Design review of the part built by this model. Coordinates are the model's own, in mm. Face numbers are marked on the shaded views. A direction names the side the tool comes from. Give positions to 0.01 mm unless a question says otherwise; leave off trailing zeros. Loops run counter-clockwise (first coordinate to the right, second up) from the corner with the lowest first, then second, coordinate; pieces in that order, holes last.
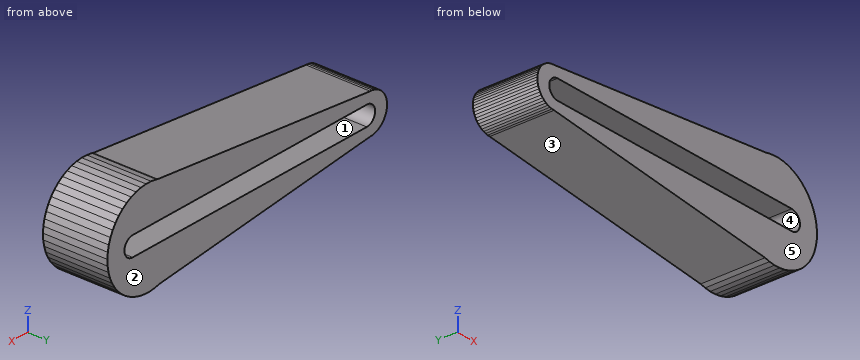
from build123d import *

# Parameters (mm, degrees)
F1_DEPTH = 25.4
F2_W     = 107.95
F2_H     = 7.62
F3_DEPTH = 25.4


with BuildPart() as f1:
    # F0 (on Front) → F1 (new body)
    with BuildSketch(Plane.XZ):
        Polygon((34.795007, 14.206795), (36.671421, 15.617947), (38.709903, 16.782795), (40.878305, 17.682968), (42.411124, 18.103591), (-55.535455, 7.733652), (-54.566239, 7.671582), (-53.612446, 7.488527), (-52.689117, 7.187373), (-51.810813, 6.77287), (-50.991386, 6.251554), (-50.243758, 5.631648), (-49.57972, 4.922928), (-49.009745, 4.13657), (-48.542821, 3.284975), (-48.186312, 2.381575), (-47.94584, 1.440616), (-47.825198, 0.476938), (-47.826288, -0.494263), (-47.949093, -1.457668), (-48.191676, -2.398085), (-48.550212, -3.300683), (-49.019046, -4.151227), (-49.590785, -4.936303), (-50.256412, -5.643531), (-51.005429, -6.261758), (-51.826025, -6.781233), (-52.705257, -7.193763), (-53.62926, -7.492844), (-54.583462, -7.673758), (-55.552814, -7.733652), (41.71096, -17.93242), (41.464741, -17.873512), (39.267833, -17.045337), (37.192046, -15.948346), (35.270117, -14.599841), (33.532356, -13.021087), (32.006168, -11.236983), (30.715621, -9.275665), (29.681069, -7.168064), (28.918828, -4.947418), (28.440918, -2.648749), (28.254875, -0.308308), (28.363635, 2.036996), (28.765482, 4.350175), (29.454078, 6.59475), (30.418564, 8.735321), (31.64373, 10.738131), (33.110254, 12.571594), align=None)
        Polygon((38.709903, 16.782795), (36.671421, 15.617947), (34.795007, 14.206795), (33.110254, 12.571594), (31.64373, 10.738131), (30.418564, 8.735321), (29.454078, 6.59475), (28.765482, 4.350175), (28.363635, 2.036996), (28.254875, -0.308308), (28.440918, -2.648749), (28.918828, -4.947418), (29.681069, -7.168064), (30.715621, -9.275665), (32.006168, -11.236983), (33.532356, -13.021087), (35.270117, -14.599841), (37.192046, -15.948346), (39.267833, -17.045337), (41.464741, -17.873512), (41.71096, -17.93242), (48.429475, -18.636902), (50.753616, -18.30427), (53.017741, -17.682968), (55.186143, -16.782795), (57.224625, -15.617947), (59.101039, -14.206795), (60.785793, -12.571594), (62.252316, -10.738131), (63.477482, -8.735321), (64.441968, -6.59475), (65.130564, -4.350175), (65.532411, -2.036996), (65.641171, 0.308308), (65.455129, 2.648749), (64.977218, 4.947418), (64.214977, 7.168064), (63.180425, 9.275665), (61.889879, 11.236983), (60.36369, 13.021087), (58.625929, 14.599841), (56.704, 15.948346), (54.628213, 17.045337), (52.431306, 17.873512), (50.147923, 18.419812), (47.814076, 18.67562), (42.411124, 18.103591), (40.878305, 17.682968), align=None)
        Polygon((43.14243, 18.30427), (42.411124, 18.103591), (47.814076, 18.67562), (45.466571, 18.636902), align=None)
        Polygon((-54.566239, 7.671582), (-55.535455, 7.733652), (-56.504807, 7.673758), (-57.459008, 7.492844), (-58.383011, 7.193763), (-59.262244, 6.781233), (-60.082839, 6.261758), (-60.831856, 5.643531), (-61.497483, 4.936303), (-62.069222, 4.151227), (-62.538056, 3.300683), (-62.896592, 2.398085), (-63.139176, 1.457668), (-63.261981, 0.494263), (-63.263071, -0.476938), (-63.142429, -1.440616), (-62.901957, -2.381575), (-62.545448, -3.284975), (-62.078524, -4.13657), (-61.508548, -4.922928), (-60.844511, -5.631648), (-60.096883, -6.251554), (-59.277456, -6.77287), (-58.399152, -7.187373), (-57.475822, -7.488527), (-56.522029, -7.671582), (-55.552814, -7.733652), (-54.583462, -7.673758), (-53.62926, -7.492844), (-52.705257, -7.193763), (-51.826025, -6.781233), (-51.005429, -6.261758), (-50.256412, -5.643531), (-49.590785, -4.936303), (-49.019046, -4.151227), (-48.550212, -3.300683), (-48.191676, -2.398085), (-47.949093, -1.457668), (-47.826288, -0.494263), (-47.825198, 0.476938), (-47.94584, 1.440616), (-48.186312, 2.381575), (-48.542821, 3.284975), (-49.009745, 4.13657), (-49.57972, 4.922928), (-50.243758, 5.631648), (-50.991386, 6.251554), (-51.810813, 6.77287), (-52.689117, 7.187373), (-53.612446, 7.488527), align=None)
        Polygon((48.429475, -18.636902), (41.71096, -17.93242), (43.748123, -18.419812), (46.08197, -18.67562), align=None)
    extrude(amount=F1_DEPTH)

    # F2 (on Front) → F3 (cut)
    with BuildSketch(Plane.XZ):
        Rectangle(F2_W, F2_H)
        with BuildLine():
            Line((-53.975, -3.81), (-53.975, 3.81))
            ThreePointArc((-53.975, 3.81), (-57.785, 0), (-53.975, -3.81))
        make_face()
        with BuildLine():
            ThreePointArc((53.975, -3.81), (57.785, 0), (53.975, 3.81))
            Line((53.975, 3.81), (53.975, -3.81))
        make_face()
    extrude(amount=F3_DEPTH, mode=Mode.SUBTRACT)


solid = f1.part
Q1. Take a section at A-A (x = 39). Give the boundary of the cut face in (y, z), plus the area to 3 significant figures.
Results:
outline: (-25.4, -17.65) - (0, -17.65) - (0, -3.81) - (-25.4, -3.81) - close; (-25.4, 3.81) - (0, 3.81) - (0, 17.74) - (-25.4, 17.74) - close
area: 705 mm2
Q2. Tool access review of the marked faces 4 and 5: name each direction out of +Z, -Z, +X, -X, +Y, -Y from which nothing blocks a thin tool from reaching the whole face with its end or side.
Results:
face 4: +Y, -Y
face 5: +Z, -Z, +X, -X, -Y
Q3. Take a section at B-B (x = -4). Give the boundary of the cut face in (y, z), plus the area to 3 significant figures.
Results:
outline: (-25.4, -13.14) - (0, -13.14) - (0, -3.81) - (-25.4, -3.81) - close; (-25.4, 3.81) - (0, 3.81) - (0, 13.19) - (-25.4, 13.19) - close
area: 475 mm2
Q4. Insertion check: pin 1 (3 mm diameter, centred on x = -15, y = -23, fed in from +Z); pin 2 (12.5 mm diameter, centred on x = 17, y = -11.5, fed in from -Z); pin 3 (6 mm diameter, centred on y = -8.5, z = -3.5, fed in from -X). Each pin has a flat end and moves straight along its axis. Give the tip position at first contact, or say it passes through.
Results:
pin 1: stops at z = 12.18
pin 2: stops at z = -16
pin 3: stops at x = -63.26
Q5. Wall thickness on line 1 (Z direction, x = -34.5, y = -3.25); line 2 (X direction, y = -21.75, z = -2); line 3 (Z direction, x = 56.5, y = -2): over which ranges is each line inside the solid? List them lowest first.
Results:
line 1: z = -9.94 to -3.81, 3.81 to 9.96
line 2: x = -63 to -57.22, 57.22 to 65.53
line 3: z = -16.03 to -2.85, 2.85 to 16.06
Q6. Draft analysis for pull direction X (two halves, no side actions). For the marked faces 1, 2 and 3, state which applies: pulls with the +X half, pulls with the -X half, needs draft (parallel to the pull), parting line crosses it, or undercut.
Results:
face 1: undercut
face 2: needs draft
face 3: pulls with the -X half
